```python
from build123d import *

# Parameters (mm, degrees)
F1_DEPTH = 30
F2_R     = 1


with BuildPart() as f1:
    # F0 (on Front) → F1 (new body)
    with BuildSketch(Plane.XZ):
        Polygon((-44.165032, 39.269094), (-44.165032, 19.269094), (-34.165032, 19.269094), (-34.165032, 39.269094), (-37.165032, 39.269094), (-37.165032, 22.269094), (-41.165032, 22.269094), (-41.165032, 37.231111), (-40.561296, 37.429221), (-41.165032, 39.269094), align=None)
    extrude(amount=F1_DEPTH)

    # F2
    f2_edges = [f1.edges().sort_by_distance(p)[0] for p in [
        (-34.165032, -15, 19.269094),
        (-34.165032, -15, 39.269094),
        (-37.165032, -15, 39.269094),
        (-44.165032, -15, 19.269094),
        (-44.165032, -15, 39.269094),
        (-41.165032, -15, 39.269094),
    ]]
    fillet(f2_edges, radius=F2_R)


solid = f1.part
```
CAD build for the part. Positions are in the model's coordinates, mm. A direction names the side the tool comes from. Give positions to 0.01 mm unless a question says otherwise; leave off trailing zeros. Write each loop counter-clockwise with the first axis right and the second up, starting at its lowest first coordinate (ties: lowest second). Pieces come first, ordered by that corner, then holes. Notation, with made-up numbers: M 6.25,18 L 22.25,18 A11 cw 22.25,30 Z; hole C 81,8.5 d6. An arc over 180 degrees is marked long. Return JSON: item names as keys, results as strings. Group by question number.
(1) Flat gauge pin, fed straight in: pin 1 Ø1.5 at (x, z) = (-39, 31) entering from -Y. Where does the tip first touch, or does it go through?
(2) 3-axis set-ups, long thin cutter, end or side, ignore diameter. For faces 1 (the face through (-41.165, -15, 30)), 2 (the face through (-44.165, -15, 29)), 3 (the face through (-36.864, -15.21, 38.984)): which of +Z, -Z, +X, -X, +Y, -Y reach the whole face in a straight line?
(3) Drill centre lines: L1, parallel to X at y = -28.5, z = 36.75; L2, parallel to Z at x = -37.75, y = -20.5; L3, parallel to Z at x = -41.75, y = -13.75. Where is each one in solid material? Low to high. Write a range as [from, to].
(4) Band-saw the part on A-A (z = 33.25). Give the cut face in (x, y).
(5) Band-saw the part on B-B (y = -27). Give the cut face in (x, z).
(6) Mould opens along X. For faces 4 (the face through (-34.47, -15.21, 19.55)), 5 (the face through (-41.5, -30, 29.4)), 6 (the face through (-39, -15, 22.269)) say: pulls with the +X half, pulls with the -X half, needs draft (parallel to the pull), parting line crosses it, or undercut.
(7) Band-saw the part on C-C (x = -37.75). Give the cut face in (y, z).
Entries:
{
 "1": {"pin 1": "passes through"},
 "2": {"face 1": "+Y, -Y", "face 2": "+Z, -Z, -X, +Y, -Y", "face 3": "+Z, +Y, -Y"},
 "3": {"L1": "x = [-44.17, -41.17], [-37.17, -34.17]", "L2": "z = [19.27, 22.27]", "L3": "z = [19.27, 39.26]"},
 "4": {"outline": "M -44.17,-30 L -41.17,-30 L -41.17,0 L -44.17,0 Z; M -37.17,-30 L -34.17,-30 L -34.17,0 L -37.17,0 Z"},
 "5": {"outline": "M -44.17,20.27 A1 ccw -43.17,19.27 L -35.17,19.27 A1 ccw -34.17,20.27 L -34.17,38.27 A1 ccw -35.17,39.27 L -36.17,39.27 A1 ccw -37.17,38.27 L -37.17,22.27 L -41.17,22.27 L -41.17,37.23 L -40.56,37.43 L -40.94,38.58 A1 ccw -41.89,39.27 L -43.17,39.27 A1 ccw -44.17,38.27 Z"},
 "6": {"face 4": "pulls with the +X half", "face 5": "needs draft", "face 6": "undercut"},
 "7": {"outline": "M -30,19.27 L 0,19.27 L 0,22.27 L -30,22.27 Z"}
}
